Print and shaded views of the part. All mm, measured from the part's lowest x, y and z. A direction names the side the tool comes from. Round coordinates to 2 decimals unless told otherwise and drop trailing zeros. Order: outer loops, then holes, each group sorted by start corner. A loop starts at its lowest first (then second) coordinate and runs counter-clockwise, first axis right, second up. Notation, with made-up numbers: (5, -12) - (26, -12) arc R14 ccw to (26, -7) - close; hole circle Ø11 at (-31.75, -10.75). An arc over 180 degrees is marked (long way). Return JSON: item names as keys, results as strings. Group by question number.
Item 1: Saw through at C-C on z = 5. List the corners of the cut face in (x, y).
Item 2: Tool access for the marked faces 1 and 2: list every direction of +Z, -Z, +X, -X, +Y, -Y with a clear straight run to the whole face (end or side of a thin tool).
Item 3: Saw through at D-D on x = 3.5. List the corners of the cut face in (y, z), and give its area (3 significant figures).
Item 4: Two-plate mould, pull along Y, no slides. Class the marked faces 3, 4, 5 and 6: released by +Y, released by -Y, zero draft, split by the parting line, or undercut.
Item 5: Probe probe 1 along Y at (x, z) = (7.5, 1.2); probe 2 along Y at (x, z) = (8.25, 2.75); probe 3 along X at (y, z) = (92.5, 1.5). List the from-to ranges inside material, lowest first.
Item 6: Saw through at B-B on y = 92.5. List the corners of the cut face in (x, z), and give its area (3 significant figures).
Item 7: Saw through at A-A on x = 7.5. List the corners of the cut face in (y, z), and give its area (3 significant figures).
Item 8: Drop flat-ended pins along their axis: pin 1 (3 mm diameter, centred on x = 7.5, y = 67.5, fed in from +Z); pin 2 (1.5 mm diameter, centred on x = 3.5, z = 6.5, fed in from -Y); pin 3 (1 mm diameter, centred on y = 18.5, z = 9.5, fed in from +X). Give the stop position or say it passes through.
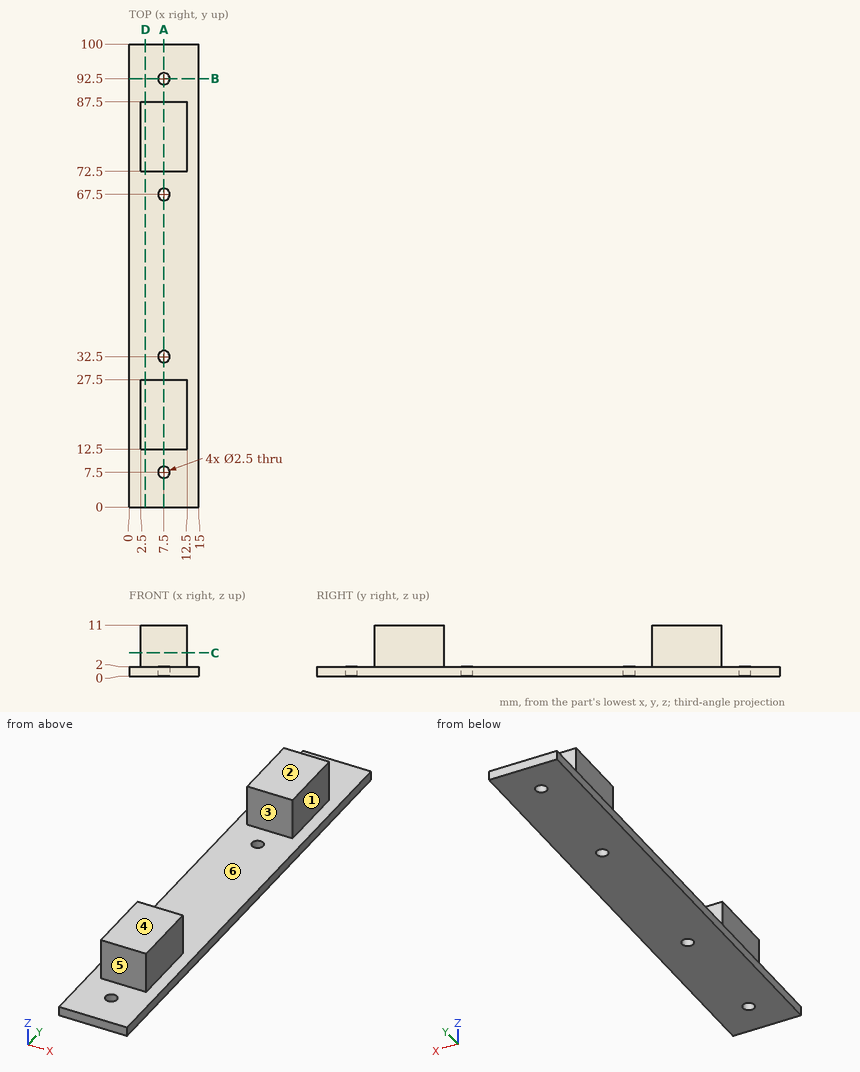
Filled in:
{
 "1": {"outline": "(2.5, 12.5) - (12.5, 12.5) - (12.5, 27.5) - (2.5, 27.5) - close; (2.5, 72.5) - (12.5, 72.5) - (12.5, 87.5) - (2.5, 87.5) - close"},
 "2": {"face 1": "+Z, +X, +Y, -Y", "face 2": "+Z, +X, -X, +Y, -Y"},
 "3": {"outline": "(0, 0) - (100, 0) - (100, 2) - (87.5, 2) - (87.5, 11) - (72.5, 11) - (72.5, 2) - (27.5, 2) - (27.5, 11) - (12.5, 11) - (12.5, 2) - (0, 2) - close", "area": "470 mm^2"},
 "4": {"face 3": "undercut", "face 4": "zero draft", "face 5": "released by -Y", "face 6": "undercut"},
 "5": {"probe 1": "y = 0 to 6.25, 8.75 to 31.25, 33.75 to 66.25, 68.75 to 91.25, 93.75 to 100", "probe 2": "y = 12.5 to 27.5, 72.5 to 87.5", "probe 3": "x = 0 to 6.25, 8.75 to 15"},
 "6": {"outline": "(0, 0) - (6.25, 0) - (6.25, 2) - (0, 2) - close; (8.75, 0) - (15, 0) - (15, 2) - (8.75, 2) - close", "area": "25.0 mm^2"},
 "7": {"outline": "(0, 0) - (6.25, 0) - (6.25, 2) - (0, 2) - close; (8.75, 0) - (31.25, 0) - (31.25, 2) - (27.5, 2) - (27.5, 11) - (12.5, 11) - (12.5, 2) - (8.75, 2) - close; (33.75, 0) - (66.25, 0) - (66.25, 2) - (33.75, 2) - close; (68.75, 0) - (91.25, 0) - (91.25, 2) - (87.5, 2) - (87.5, 11) - (72.5, 11) - (72.5, 2) - (68.75, 2) - close; (93.75, 0) - (100, 0) - (100, 2) - (93.75, 2) - close", "area": "450 mm^2"},
 "8": {"pin 1": "stops at z = 2", "pin 2": "stops at y = 12.5", "pin 3": "stops at x = 12.5"}
}
